from build123d import *

# Parameters (mm, degrees)
SKETCH006_R            = 2.3495
PAD006_DEPTH           = 6.35
SKETCH007_W            = 6.35
SKETCH007_H            = 12.7
POCKET002_DEPTH        = 0.001
POCKET002_DEPTH_BACK   = 6.351
LINEARPATTERN002_COUNT = 3
LINEARPATTERN002_PITCH = 25.4
SKETCH009_W            = 6.35
SKETCH009_H            = 12.7
POCKET003_DEPTH        = 0.001
POCKET003_DEPTH_BACK   = 6.351
LINEARPATTERN003_COUNT = 3
LINEARPATTERN003_PITCH = 25.4


with BuildPart() as part:
    # Sketch006 → Pad006 (new body)
    with BuildSketch(Plane.XZ):
        with BuildLine():
            Line((533.4, 6.35), (533.4, 76.2))
            Line((533.4, 76.2), (66.675, 76.2))
            ThreePointArc((63.5, 79.375), (64.429936, 77.129936), (66.675, 76.2))
            Line((63.5, 79.375), (63.5, 101.6))
            Line((63.5, 101.6), (6.35, 101.6))
            Line((6.35, 101.6), (6.35, 82.55))
            Line((6.35, 82.55), (0, 82.55))
            Line((0, 82.55), (0, 6.35))
            Line((0, 6.35), (533.4, 6.35))
        make_face()
        with Locations((508, 63.5)):
            Circle(SKETCH006_R, mode=Mode.SUBTRACT)
        with Locations((508, 19.05)):
            Circle(SKETCH006_R, mode=Mode.SUBTRACT)
        with Locations((25.4, 19.05)):
            Circle(SKETCH006_R, mode=Mode.SUBTRACT)
        with Locations((25.4, 88.9)):
            Circle(SKETCH006_R, mode=Mode.SUBTRACT)
    extrude(amount=PAD006_DEPTH)

    # Sketch007 → Pocket002 (cut, two sides)
    with BuildSketch(Plane.XZ) as pocket002_sk:
        with Locations((3.175, 12.7)):
            Rectangle(SKETCH007_W, SKETCH007_H)
    pocket002 = extrude(amount=-POCKET002_DEPTH, mode=Mode.SUBTRACT) + extrude(pocket002_sk.sketch, amount=POCKET002_DEPTH_BACK, mode=Mode.SUBTRACT)

    # LinearPattern002: Pocket002 ×3
    with Locations(*[(0, 0, i * LINEARPATTERN002_PITCH) for i in range(1, LINEARPATTERN002_COUNT)]):
        add(pocket002, mode=Mode.SUBTRACT)

    # Sketch009 → Pocket003 (cut, two sides)
    with BuildSketch(Plane.XZ) as pocket003_sk:
        with Locations((530.225, 12.7)):
            Rectangle(SKETCH009_W, SKETCH009_H)
    pocket003 = extrude(amount=-POCKET003_DEPTH, mode=Mode.SUBTRACT) + extrude(pocket003_sk.sketch, amount=POCKET003_DEPTH_BACK, mode=Mode.SUBTRACT)

    # LinearPattern003: Pocket003 ×3
    with Locations(*[(0, 0, i * LINEARPATTERN003_PITCH) for i in range(1, LINEARPATTERN003_COUNT)]):
        add(pocket003, mode=Mode.SUBTRACT)


solid = part.part
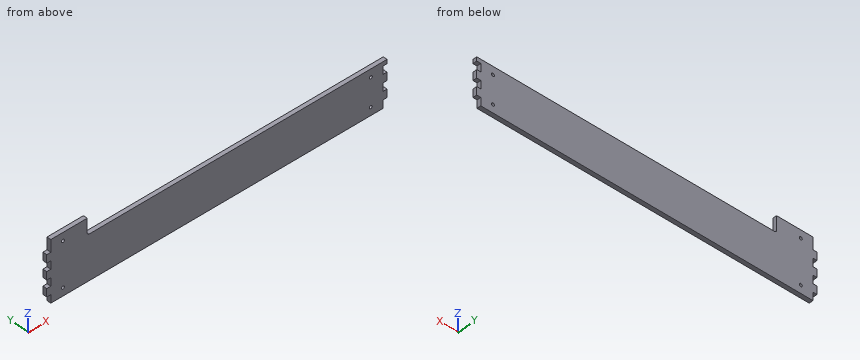
Can you work these out from the model? Positions are in its coordinate system, mm. Give positions to 0.01 mm unless a question says otherwise; leave off trailing zeros. Order: outer loops, then holes, each group sorted by start corner. A loop starts at its lowest first (then second) coordinate and runs counter-clockwise, first axis right, second up. Notation, with made-up numbers: M 19.5,-19.5 L 58.5,-19.5 A27 cw 58.5,18.5 Z; hole C 23,-7.75 d5. An arc over 180 degrees is marked long. One line per item, written item: value.
Item 1: Please list where these lines run through material, in increasing order: line 1 (Z direction, x = 508, y = -4.5); line 2 (Z direction, x = 25.4, y = -3.25); line 3 (Z direction, x = 323, y = -2.75).
Verdict:
line 1: 6.35 to 16.7, 21.4 to 61.15, 65.85 to 76.2
line 2: 6.35 to 16.7, 21.4 to 86.55, 91.25 to 101.6
line 3: 6.35 to 76.2
Item 2: If we section it at B-B on x = 130: Write out the boundary of the cut face in (y, z).
Verdict:
outline: M -6.35,6.35 L 0,6.35 L 0,76.2 L -6.35,76.2 Z
Item 3: If we section it at A-A on y = -5.25: State how many separate pieces and enclosed holes the cut face has, and give its area (3 significant figures).
Verdict:
separate pieces: 1
enclosed holes: 4
area: 38,200 mm2
Item 4: For pin 1 (1.9 mm diameter, centred on x = 529, y = -4, fed in from -Z); pin 2 (6 mm diameter, centred on x = 508, z = 19.05, fed in from -Y); pin 3 (2 mm diameter, centred on y = -5.5, z = 63.5, fed in from -X); pin 4 (3 mm diameter, centred on y = -4.5, z = 37, fed in from +X), each with a flat end and sliding along its axis, tell me the tip position at first contact or that it passes through.
Verdict:
pin 1: z = 19.05
pin 2: y = -6.35
pin 3: x = 6.35
pin 4: x = 527.05
